Input: dimensioned drawing with shaded views. Units: mm. Origin: part minimum x, y, z. A direction names the side the tool comes from. Round coordinates to 2 decimals unless told otherwise and drop trailing zeros. Order: outer loops, then holes, each group sorted by start corner. A loop starts at its lowest first (then second) coordinate and runs counter-clockwise, first axis right, second up. Notation, with made-up numbers: (-0.5, 37) - (54.5, 37) arc R22 ccw to (54.5, 68) - close; hole circle Ø11 at (-33.5, 56). An arc over 180 degrees is marked (long way). Return JSON: item names as keys, results as strings. Group by question number.
1) Ray query, line 1 (Z direction, x = 14.25, y = 5.5); line 2 (X direction, y = 7.5, z = 95.5); line 3 (Z direction, x = 8.25, y = 2.75). Return the intervals inside material, ascending. Write a range as from..to.
2) Section A-A, the plane y = 7.5. Return loops of the section in (x, z), plus the area to 3 significant figures.
3) Section C-C, the plane z = 54.5. Return loops of the section in (x, y), plus the area to 3 significant figures.
4) Contact query for flat-ended pins moving along their axis: P1, Ø3, axis at y = 8, z = 107, coming from the -X side; P2, Ø6, axis at y = 4, z = 57, coming from the +X side; P3, Ø4.5, axis at y = 7.5, z = 105.5, coming from the +X side. Output: stop coordinate, or through.
5) Section B-B, the plane x = 7.5. Return loops of the section in (y, z), plus the area to 3 significant figures.
6) Access query for the marked faces 1 and 2. Directions: +Z, -Z, +X, -X, +Y, -Y. A direction counts if a zero-diameter tool reaches every point of the face in a straight line with its end or side. Return the directions, or none.
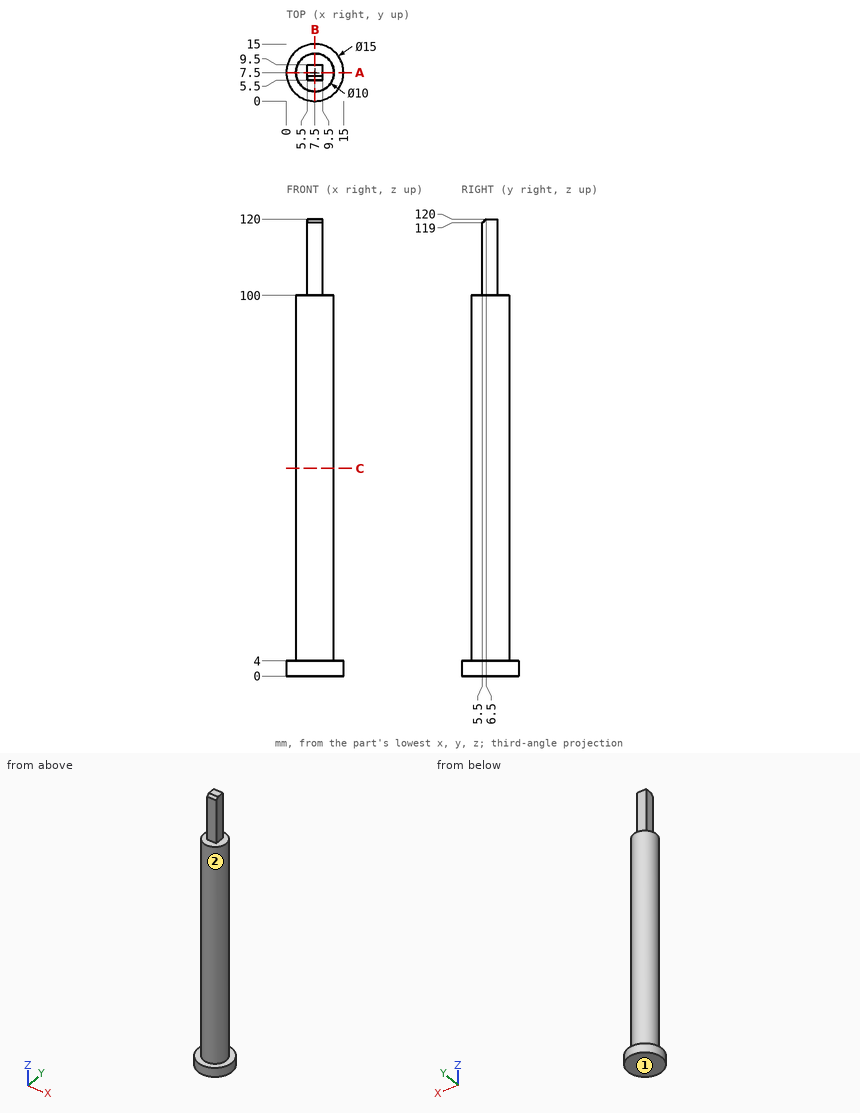
Geometry check:
{
 "1": {"line 1": "0..4", "line 2": "2.5..12.5", "line 3": "0..100"},
 "2": {"outline": "(0, 0) - (15, 0) - (15, 4) - (12.5, 4) - (12.5, 100) - (9.5, 100) - (9.5, 120) - (5.5, 120) - (5.5, 100) - (2.5, 100) - (2.5, 4) - (0, 4) - close", "area": "1,100 mm2"},
 "3": {"outline": "circle Ø10 at (7.5, 7.5)", "area": "78.5 mm2"},
 "4": {"P1": "x = 5.5", "P2": "x = 12.47", "P3": "x = 9.5"},
 "5": {"outline": "(0, 0) - (15, 0) - (15, 4) - (12.5, 4) - (12.5, 100) - (9.5, 100) - (9.5, 120) - (6.5, 120) - (5.5, 119) - (5.5, 100) - (2.5, 100) - (2.5, 4) - (0, 4) - close", "area": "1,100 mm2"},
 "6": {"face 1": "-Z, +X, -X, +Y, -Y", "face 2": "+Z"}
}
